Check sheet for the drawn part. Datum: minimum x, y, z corner. Units: mm. A direction names the side the tool comes from. Round coordinates to 2 decimals unless told otherwise and drop trailing zeros. Order: outer loops, then holes, each group sorted by start corner. A loop starts at its lowest first (then second) coordinate and runs counter-clockwise, first axis right, second up. Notation, with made-up numbers: (-6, 12) -> (15, 12) arc R21 cw to (15, 50) -> close; hole circle Ø11 at (-12, 60.25). An arc over 180 degrees is marked (long way). Answer as a JSON object with one key per item and string values. Group by question number.
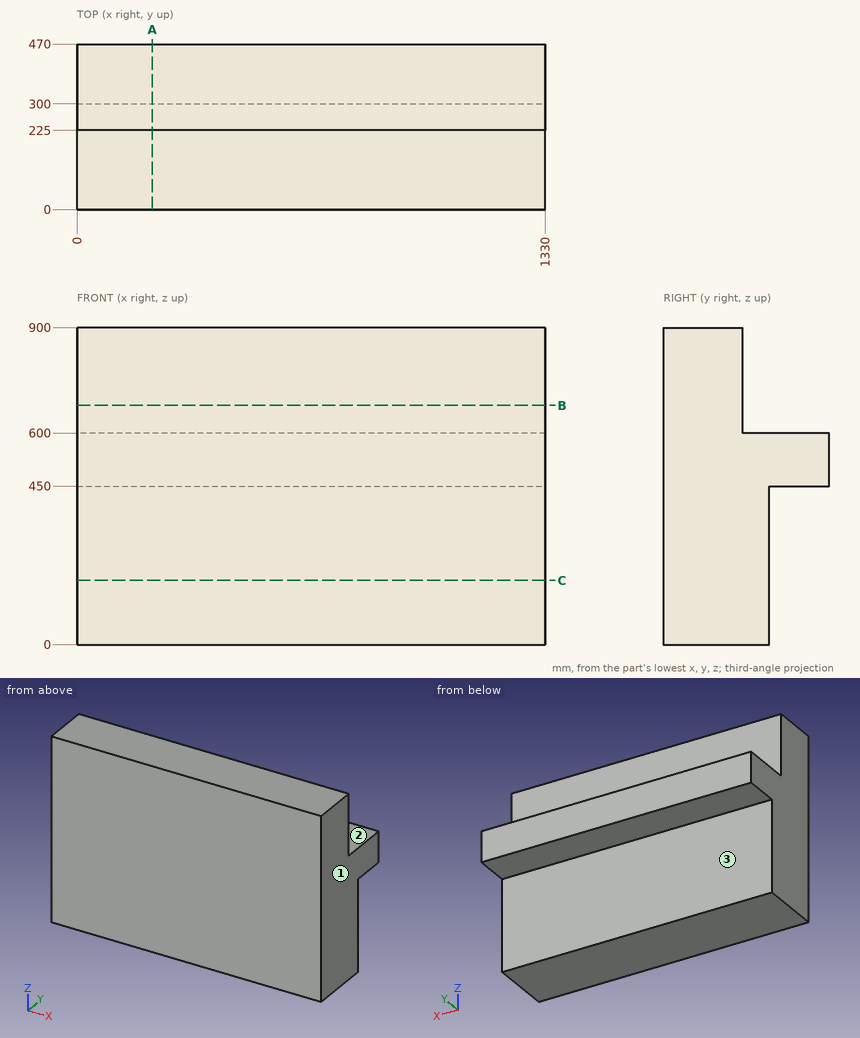
Item 1: Thickness scan on L1, parallel to Y at x = 122, z = 40.5; L2, parallel to Y at x = 717, z = 715; L3, parallel to Z at x = 94, y = 296. Record the ranges inside material, lowest first.
Item 2: Depth check by flat-ended pin: pin 1 Ø1 at (x, z) = (906, 733) entering from +Y. Enter the tip coordinate at first touch or a pass-through.
Item 3: Sectioned sample at B-B, the plane z = 679. Enter the section's corners in (x, y), then the cut area to 3 significant figures.
Item 4: Sectioned sample at C-C, the plane z = 182. Enter the section's corners in (x, y), then the cut area to 3 significant figures.
Item 5: Sectioned sample at A-A, the plane x = 214. Enter the section's corners in (y, z), then the cut area to 3 significant figures.
Item 6: Set-up check for the marked faces 1, 2 and 3: record each of +Z, -Z, +X, -X, +Y, -Y from which the full face is reachable in a straight line by a thin tool's end or side.
Result:
{
 "1": {"L1": "y = 0 to 300", "L2": "y = 0 to 225", "L3": "z = 0 to 600"},
 "2": {"pin 1": "stops at y = 225"},
 "3": {"outline": "(0, 0) -> (1330, 0) -> (1330, 225) -> (0, 225) -> close", "area": "299,000 mm2"},
 "4": {"outline": "(0, 0) -> (1330, 0) -> (1330, 300) -> (0, 300) -> close", "area": "399,000 mm2"},
 "5": {"outline": "(0, 0) -> (300, 0) -> (300, 450) -> (470, 450) -> (470, 600) -> (225, 600) -> (225, 900) -> (0, 900) -> close", "area": "273,000 mm2"},
 "6": {"face 1": "+Z, -Z, +X, +Y, -Y", "face 2": "+Z, +X, -X, +Y", "face 3": "-Z, +X, -X, +Y"}
}
